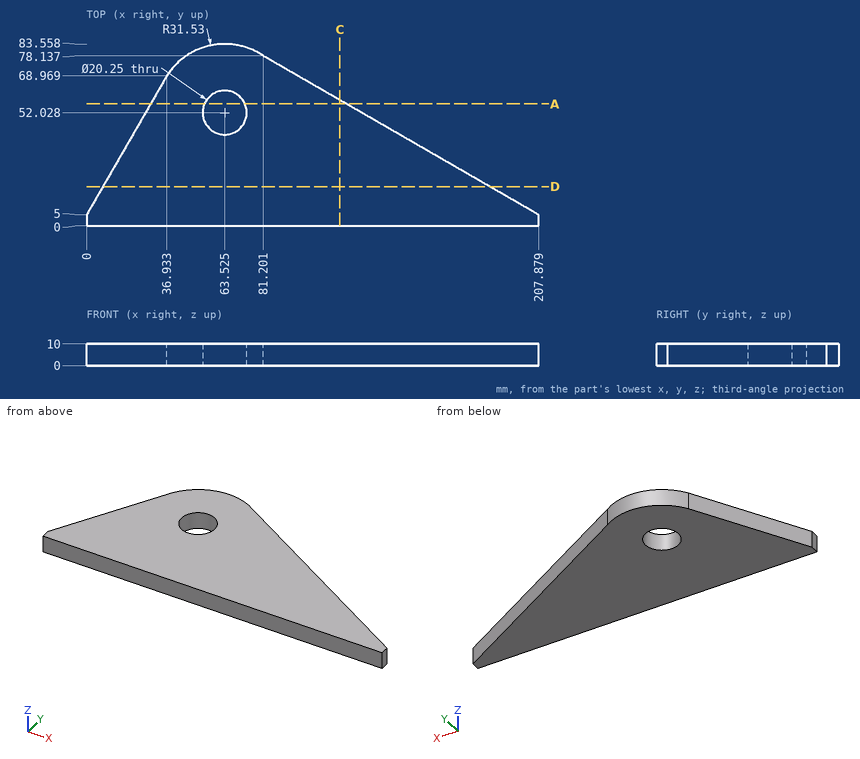
Part print with two shaded views. Sizes in mm from the minimum x, y, z corner. Coordinates: 2 decimals unless noted, no trailing zeros. Order: outer loops, then holes, each group sorted by start corner. A loop starts at its lowest first (then second) coordinate and runs counter-clockwise, first axis right, second up.
(1) Drill centre lines: L1, parallel to Y at x = 57.5, z = 3 (1 decimal); L2, parallel to X at y = 50.5, z = 7 (1 decimal); L3, parallel to X at y = 47.5, z = 3 (1 decimal). Where is each one in solid material? Low to high.
Solution:
L1: y = 0 to 43.9, 60.2 to 83
L2: x = 26.3 to 53.5, 73.5 to 129.1
L3: x = 24.5 to 54.5, 72.6 to 134.3
(2) Saw through at C-C, the plane x = 116.5. Write the cut outline in (y, z).
Solution:
outline: (0, 0) - (57.76, 0) - (57.76, 10) - (0, 10) - close
(3) Pin check, flat tips, straight feed: pin 1 Ø6 at (y, z) = (60, 7.5) entering from -X; pin 2 Ø3 at (y, z) = (33.5, 7.5) entering from +X (1 decimal); pin 3 Ø3 at (x, y) = (116, 44.5) entering from -Z; pin 4 Ø5 at (y, z) = (26, 1) entering from -X. Stop position of each tip, or through.
Solution:
pin 1: stops at x = 30.02
pin 2: stops at x = 161.1
pin 3: stops at z = 0
pin 4: stops at x = 10.68
(4) Saw through at A-A, the plane y = 56. Write the cut outline in (x, z) (1 decimal).
Solution:
outline: (29.4, 0) - (54.2, 0) - (54.2, 10) - (29.4, 10) - close; (72.8, 0) - (119.5, 0) - (119.5, 10) - (72.8, 10) - close
(5) Saw through at D-D, the plane y = 18. Write the cut outline in (x, z) (1 decimal), and give its area (3 significant figures).
Solution:
outline: (7.5, 0) - (185.4, 0) - (185.4, 10) - (7.5, 10) - close
area: 1,780 mm2
